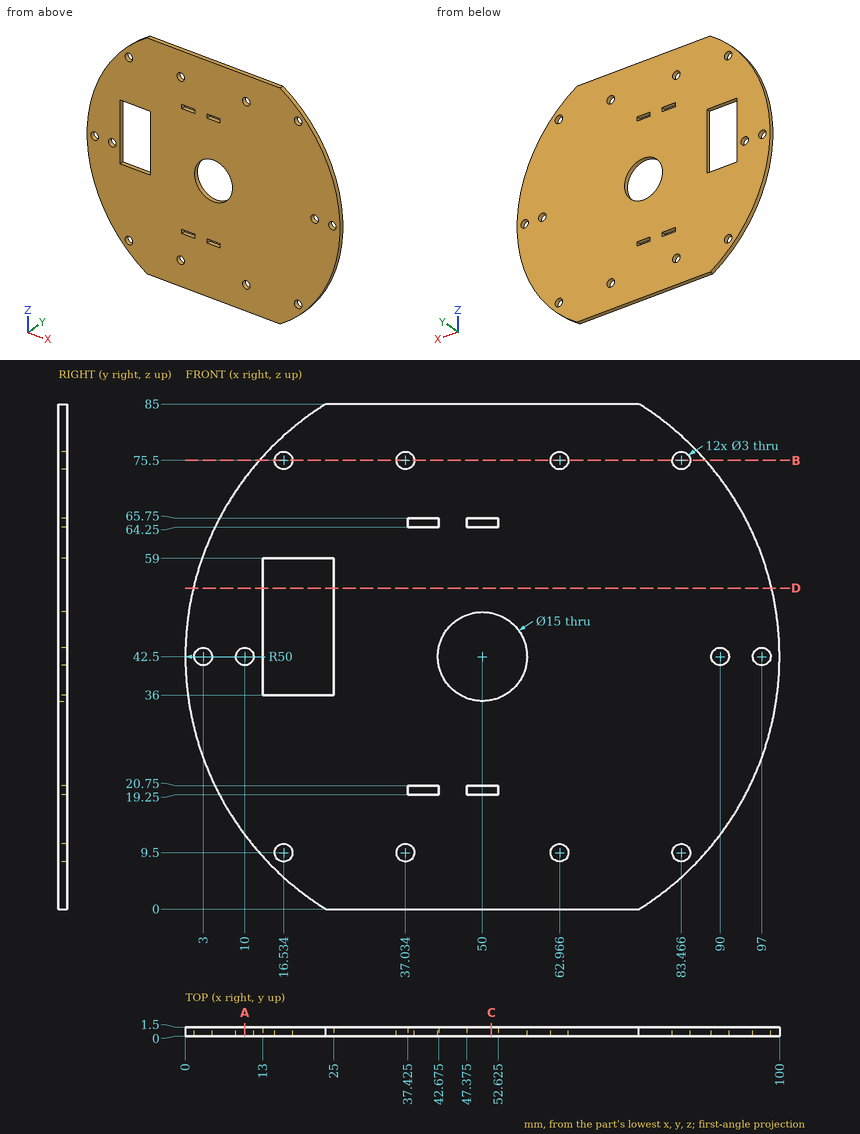
Verification items for this drawing (mm, ordinates from the low corner). Round coordinates to 2 decimals unless told otherwise and drop trailing zeros. Loops run counter-clockwise (first coordinate to the right, second up) from the corner with the lowest first, then second, coordinate; pieces in that order, holes last. Notation, with made-up numbers: (26, -6.5) -> (35, -6.5) arc R17 cw to (35, 23.5) -> close; hole circle Ø3 at (-16, 64). An arc over 180 degrees is marked (long way). Write item = value, one per line. Start each with the question number.
1) Sectioned sample at A-A, the plane x = 10. Record the cut outline in (y, z).
2) Sectioned sample at D-D, the plane z = 54. Record the cut outline in (x, y).
3) Sectioned sample at C-C, the plane x = 51.5. Record the cut outline in (y, z), plus the area to 3 significant figures.
4) Gauge pin test, flat ends, axial feed: pin 1 Ø0.8 at (y, z) = (0.5, 65.5) entering from -X; pin 2 Ø0.8 at (y, z) = (0.5, 50.5) entering from -X; pin 3 Ø2.5 at (x, z) = (37.03, 9.5) entering from +Y. Record the tip position at first contact, or that the pin passes through.
5) Thickness scan on probe 1 along X at (y, z) = (1.2, 9.5) (1 decimal); probe 2 along X at (y, z) = (1.15, 45); probe 3 along Z at (x, y) = (17, 0.35) (1 decimal). Record the ranges inside material, lowest first.
6) Sectioned sample at B-B, the plane z = 75.5. Record the cut outline in (x, y).
Results are:
q1.outline = (0, 12.5) -> (1.5, 12.5) -> (1.5, 41) -> (0, 41) -> close; (0, 44) -> (1.5, 44) -> (1.5, 72.5) -> (0, 72.5) -> close
q2.outline = (1.34, 0) -> (13, 0) -> (13, 1.5) -> (1.34, 1.5) -> close; (25, 0) -> (98.66, 0) -> (98.66, 1.5) -> (25, 1.5) -> close
q3.outline = (0, 0) -> (1.5, 0) -> (1.5, 19.25) -> (0, 19.25) -> close; (0, 20.75) -> (1.5, 20.75) -> (1.5, 35.15) -> (0, 35.15) -> close; (0, 49.85) -> (1.5, 49.85) -> (1.5, 64.25) -> (0, 64.25) -> close; (0, 65.75) -> (1.5, 65.75) -> (1.5, 85) -> (0, 85) -> close
q3.area = 101 mm^2
q4.pin_1 = 5.4
q4.pin_2 = 0.58
q4.pin_3 = through
q5.probe_1 = 12.4 to 15, 18 to 35.5, 38.5 to 61.5, 64.5 to 82, 85 to 87.6
q5.probe_2 = 0.06 to 13, 25 to 42.93, 57.07 to 99.94
q5.probe_3 = 4.9 to 8.1, 10.9 to 36, 59 to 74.1, 76.9 to 80.1
q6.outline = (12.44, 0) -> (15.03, 0) -> (15.03, 1.5) -> (12.44, 1.5) -> close; (18.03, 0) -> (35.53, 0) -> (35.53, 1.5) -> (18.03, 1.5) -> close; (38.53, 0) -> (61.47, 0) -> (61.47, 1.5) -> (38.53, 1.5) -> close; (64.47, 0) -> (81.97, 0) -> (81.97, 1.5) -> (64.47, 1.5) -> close; (84.97, 0) -> (87.56, 0) -> (87.56, 1.5) -> (84.97, 1.5) -> close
